```python
from build123d import *

# Parameters (mm, degrees)
SKETCH1_W           = 148
SKETCH1_H           = 148
BOSS_EXTRUDE1_DEPTH = 12.7
SKETCH2_W           = 10.53028371
SKETCH2_H           = 7.9375
CUT_EXTRUDE1_DEPTH  = 12.7
SKETCH4_W           = 10
SKETCH4_H           = 5
CUT_EXTRUDE2_DEPTH  = 13.7
CIRPATTERN1_COUNT   = 4


with BuildPart() as part:
    # Sketch1 → Boss-Extrude1 (new body)
    with BuildSketch(Plane(origin=(0, 0, 0), x_dir=(1, 0, 0), z_dir=(0, 1, 0))):
        with Locations((74, 74)):
            Rectangle(SKETCH1_W, SKETCH1_H)
    extrude(amount=BOSS_EXTRUDE1_DEPTH)

    # Sketch2 → Cut-Extrude1 (cut)
    with BuildSketch(Plane(origin=(0, 12.7, 0), x_dir=(1, 0, 0), z_dir=(0, 1, 0))):
        with BuildLine():
            ThreePointArc((79.265141855, 81.9375), (82.392737967, 78.504173), (83.525, 74))
            Line((83.525, 74), (83.525, 89.875))
            Line((83.525, 89.875), (64.475, 89.875))
            Line((64.475, 89.875), (64.475, 74))
            ThreePointArc((64.475, 74), (65.607262033, 78.504173), (68.734858145, 81.9375))
            ThreePointArc((68.734858145, 81.9375), (74, 83.525), (79.265141855, 81.9375))
        make_face()
        with BuildLine():
            ThreePointArc((79.265141855, 66.0625), (82.392737967, 69.495827), (83.525, 74))
            Line((83.525, 74), (79.265141855, 74))
            Line((79.265141855, 74), (79.265141855, 66.0625))
        make_face()
        with BuildLine():
            Line((79.265141855, 74), (83.525, 74))
            ThreePointArc((83.525, 74), (82.392737967, 78.504173), (79.265141855, 81.9375))
            Line((79.265141855, 81.9375), (79.265141855, 74))
        make_face()
        with BuildLine():
            Line((68.734858145, 66.0625), (68.734858145, 74))
            Line((68.734858145, 74), (64.475, 74))
            ThreePointArc((64.475, 74), (65.607262033, 69.495827), (68.734858145, 66.0625))
        make_face()
        with BuildLine():
            Line((64.475, 74), (68.734858145, 74))
            Line((68.734858145, 74), (68.734858145, 81.9375))
            ThreePointArc((68.734858145, 81.9375), (65.607262033, 78.504173), (64.475, 74))
        make_face()
        with Locations((74, 77.96875)):
            Rectangle(SKETCH2_W, SKETCH2_H)
        with BuildLine():
            Line((68.734858145, 81.9375), (79.265141855, 81.9375))
            ThreePointArc((79.265141855, 81.9375), (74, 83.525), (68.734858145, 81.9375))
        make_face()
        with Locations((74, 70.03125)):
            Rectangle(SKETCH2_W, SKETCH2_H)
    extrude(amount=-CUT_EXTRUDE1_DEPTH, mode=Mode.SUBTRACT)

    # Sketch4 → Cut-Extrude2 (cut, through all)
    with BuildSketch(Plane(origin=(0, 12.7, 0), x_dir=(1, 0, 0), z_dir=(0, 1, 0))):
        with Locations((148, 74)):
            Rectangle(SKETCH4_W, SKETCH4_H)
    cut_extrude2 = extrude(amount=-CUT_EXTRUDE2_DEPTH, mode=Mode.SUBTRACT)

    # CirPattern1: Cut-Extrude2 ×4 about axis
    cirpattern1_axis = Axis((73.916648848, 0, -73.910393573), (0, 1, 0))
    for i in range(1, CIRPATTERN1_COUNT):
        add(cut_extrude2.rotate(cirpattern1_axis, i * 360 / CIRPATTERN1_COUNT), mode=Mode.SUBTRACT)


solid = part.part
```
Here's how the part is built. I have some questions about the finished solid (model axes, mm). A direction names the side the tool comes from. Round coordinates to 2 decimals unless told otherwise and drop trailing zeros. Loops run counter-clockwise (first coordinate to the right, second up) from the corner with the lowest first, then second, coordinate; pieces in that order, holes last.
1. Will these pins go through, and if not, where does the flat tip stop? pin 1 (6 mm diameter, centred on x = 102.5, y = 11, fed in from +Z); pin 2 (2.5 mm diameter, centred on y = 4.5, z = -74.5, fed in from -X).
Answers:
pin 1: stops at z = 0
pin 2: stops at x = 4.83
2. Suppose I cut it at A-A, the plane z = -83.5. Please give me the cut outline in (x, y) (3 decimals).
Answers:
outline: (0, 0) - (64.475, 0) - (64.475, 12.7) - (0, 12.7) - close; (83.525, 0) - (148, 0) - (148, 12.7) - (83.525, 12.7) - close
3. For faces 5 (the face through (143, 6, -74)), 6 (the face through (64.475, 6, -82)), 7 (the face through (71.506, 6, -2)), which set-ups out of +Z, -Z, +X, -X, +Y, -Y let a thin tool reach every point of the face, with its end or its side?
Answers:
face 5: +X, +Y, -Y
face 6: +Y, -Y
face 7: +Z, +Y, -Y
4. If I drill on probe 1 along Z at (x, y) = (72.5, 8) (1 decimal); probe 2 along X at (y, z) = (7.5, -72); probe 3 along X at (y, z) = (9.5, -70.5), over which ranges is the centre line in solid material (lowest first)?
Answers:
probe 1: z = -143 to -89.9, -66.1 to -4.8
probe 2: x = 4.83 to 64.69, 83.31 to 143
probe 3: x = 0 to 65.14, 82.86 to 148
5. Thinking about a two-plate mould opening in X: for faces 1 (the face through (2, 6, -71.321)), 2 (the face through (0, 6, -112)), 3 (the face through (76.506, 6, -2)), 4 (the face through (74, 6, -89.875)), which applies, released by +X, released by -X, zero draft, split by the parting line, or undercut?
Answers:
face 1: zero draft
face 2: released by -X
face 3: undercut
face 4: undercut
